from build123d import *

# Parameters (mm, degrees)
BOSS_EXTRUDE1_DEPTH = 10.16
FILLET1_R           = 19.05
SKETCH2_W           = 120.284747719
SKETCH2_H           = 20.32
SKETCH2_W_2         = 102.891608588
CUT_EXTRUDE1_DEPTH  = 12.7
SKETCH6_R           = 6.35
CUT_EXTRUDE2_DEPTH  = 10.16


with BuildPart() as part:
    # Sketch1 → Boss-Extrude1 (new body)
    with BuildSketch(Plane.XY):
        Polygon((-288.275887252, 0), (-215.032557346, 1054.1), (215.032557346, 1054.1), (288.275887252, 0), (596.950713016, 0), (596.950713016, 20.32), (457.769290722, 178.8375841), (368.537470958, 1463.04), (215.892500906, 1463.04), (-205.715298803, 1463.040000035), (-647.718210796, 1463.04), (-647.718210796, 0), align=None)
        Polygon((-609.618210796, 127), (-609.618210796, 461.510956689), (-365.626284392, 127), align=None, mode=Mode.SUBTRACT)
        Polygon((-609.618210796, 592.582701044), (-609.618210796, 907.626666667), (-314.736774564, 907.626666667), align=None, mode=Mode.SUBTRACT)
        Polygon((-282.735998162, 867.476761947), (-304.419486117, 555.413333333), (-574.827649063, 555.413333333), align=None, mode=Mode.SUBTRACT)
        Polygon((-307.949285149, 504.613333333), (-331.453012037, 166.353473425), (-578.179384354, 504.613333333), align=None, mode=Mode.SUBTRACT)
        Polygon((-609.618210796, 958.426666667), (-609.618210796, 1288.067621407), (-310.704175954, 958.426666667), align=None, mode=Mode.SUBTRACT)
        Polygon((-575.330448642, 1325.88), (-250.884200804, 1325.88), (-273.976047339, 993.547820907), align=None, mode=Mode.SUBTRACT)
        Polygon((19.05, 1104.9), (19.05, 1368.504716774), (182.716004616, 1104.9), align=None, mode=Mode.SUBTRACT)
        Polygon((41.473134849, 1404.62), (184.313325179, 1404.62), (202.313466912, 1145.566384812), align=None, mode=Mode.SUBTRACT)
        Polygon((-184.313325179, 1404.62), (-41.473134849, 1404.62), (-202.313466912, 1145.566384812), align=None, mode=Mode.SUBTRACT)
        Polygon((-19.05, 1368.504716774), (-19.05, 1104.9), (-182.716004616, 1104.9), align=None, mode=Mode.SUBTRACT)
    extrude(amount=BOSS_EXTRUDE1_DEPTH)

    # Fillet1
    fillet1_edges = [part.edges().sort_by_distance(p)[0] for p in [
        (19.05, 1368.504716774, 5.08),
        (19.05, 1104.9, 5.08),
        (182.716004616, 1104.9, 5.08),
        (-250.884200804, 1325.88, 5.08),
        (-575.330448642, 1325.88, 5.08),
        (-273.976047339, 993.547820907, 5.08),
        (-647.718210796, 1463.04, 5.08),
        (368.537470958, 1463.04, 5.08),
        (457.769290722, 178.8375841, 5.08),
        (215.032557346, 1054.1, 5.08),
        (-215.032557346, 1054.1, 5.08),
        (-609.618210796, 1288.067621407, 5.08),
        (-609.618210796, 958.426666667, 5.08),
        (-310.704175954, 958.426666667, 5.08),
        (-609.618210796, 461.510956689, 5.08),
        (-609.618210796, 127, 5.08),
        (-365.626284392, 127, 5.08),
        (-41.473134849, 1404.62, 5.08),
        (-184.313325179, 1404.62, 5.08),
        (-202.313466912, 1145.566384812, 5.08),
        (-182.716004616, 1104.9, 5.08),
        (-19.05, 1104.9, 5.08),
        (-19.05, 1368.504716774, 5.08),
        (184.313325179, 1404.62, 5.08),
        (41.473134849, 1404.62, 5.08),
        (202.313466912, 1145.566384812, 5.08),
        (-578.179384354, 504.613333333, 5.08),
        (-331.453012037, 166.353473425, 5.08),
        (-307.949285149, 504.613333333, 5.08),
        (-609.618210796, 907.626666667, 5.08),
        (-609.618210796, 592.582701044, 5.08),
        (-314.736774564, 907.626666667, 5.08),
        (-574.827649063, 555.413333333, 5.08),
        (-304.419486117, 555.413333333, 5.08),
        (-282.735998162, 867.476761947, 5.08),
    ]]
    fillet(fillet1_edges, radius=FILLET1_R)

    # Sketch2 → Cut-Extrude1 (cut)
    with BuildSketch(Plane.XY.offset(10.16)):
        with Locations((-467.291089218, 10.16)):
            Rectangle(SKETCH2_W, SKETCH2_H)
        with Locations((442.613300134, 10.16)):
            Rectangle(SKETCH2_W_2, SKETCH2_H)
        Polygon((211.92306481, 1373.664189215), (222.040744894, 1374.366931824), (215.881789204, 1463.040000035), (205.715298803, 1463.040000035), align=None)
        Polygon((234.358656272, 1197.020795404), (227.836927701, 1290.916856945), (217.719247617, 1290.214114336), (224.240976188, 1196.318052795), align=None)
        Polygon((246.676567651, 1019.674658983), (240.15668194, 1113.544188093), (230.039001856, 1112.841445484), (236.558887567, 1018.971916374), align=None)
        Polygon((258.99447903, 842.328522563), (252.476436179, 936.171519242), (242.358756095, 935.468776633), (248.876798945, 841.625779953), align=None)
        Polygon((271.312390408, 664.982386142), (264.796190418, 758.798850391), (254.678510334, 758.096107781), (261.194710324, 664.279643533), align=None)
        Polygon((283.630301787, 487.636249721), (277.115944656, 581.426181539), (266.998264572, 580.72343893), (273.512621703, 486.933507112), align=None)
        Polygon((295.948213166, 310.290113301), (289.435698895, 404.053512688), (279.318018811, 403.350770078), (285.830533081, 309.587370692), align=None)
        Polygon((308.266124544, 132.94397688), (301.755453134, 226.680843836), (291.63777305, 225.978101227), (298.14844446, 132.241234271), align=None)
        Polygon((-301.755453134, 226.680843836), (-308.266124544, 132.94397688), (-298.14844446, 132.241234271), (-291.63777305, 225.978101227), align=None)
        Polygon((-289.435698895, 404.053512688), (-295.948213166, 310.290113301), (-285.830533081, 309.587370692), (-279.318018811, 403.350770078), align=None)
        Polygon((-277.115944656, 581.426181539), (-283.630301787, 487.636249721), (-273.512621703, 486.933507112), (-266.998264572, 580.72343893), align=None)
        Polygon((-264.796190418, 758.798850391), (-271.312390408, 664.982386142), (-261.194710324, 664.279643533), (-254.678510334, 758.096107781), align=None)
        Polygon((-252.476436179, 936.171519242), (-258.99447903, 842.328522563), (-248.876798945, 841.625779953), (-242.358756095, 935.468776633), align=None)
        Polygon((-240.15668194, 1113.544188093), (-246.676567651, 1019.674658983), (-236.558887567, 1018.971916374), (-230.039001856, 1112.841445484), align=None)
        Polygon((-227.836927701, 1290.916856945), (-234.358656272, 1197.020795404), (-224.240976188, 1196.318052795), (-217.719247617, 1290.214114336), align=None)
        Polygon((-222.040744894, 1374.366931824), (-211.92306481, 1373.664189215), (-205.715298803, 1463.040000035), (-215.881789204, 1463.040000035), align=None)
    extrude(amount=-CUT_EXTRUDE1_DEPTH, mode=Mode.SUBTRACT)

    # Sketch6 → Cut-Extrude2 (cut)
    with BuildSketch(Plane.XY.offset(10.16)):
        with Locations((357.1875, 1397)):
            Circle(SKETCH6_R)
        with Locations((357.1875, 1320.8)):
            Circle(SKETCH6_R)
        with Locations((304.8, 1320.8)):
            Circle(SKETCH6_R)
        with Locations((304.8, 1397)):
            Circle(SKETCH6_R)
        with Locations((382.5875, 105.41)):
            Circle(SKETCH6_R)
        with Locations((382.5875, 29.21)):
            Circle(SKETCH6_R)
        with Locations((330.2, 29.21)):
            Circle(SKETCH6_R)
        with Locations((330.2, 105.41)):
            Circle(SKETCH6_R)
        with Locations((350.023844044, 410.21)):
            Circle(SKETCH6_R)
        with Locations((346.838891066, 562.61)):
            Circle(SKETCH6_R)
    extrude(amount=-CUT_EXTRUDE2_DEPTH, mode=Mode.SUBTRACT)


solid = part.part
Read the model definition and answer for the solid it produces. Units are mm, in the model's axes. A direction names the side the tool comes from. Round coordinates to 2 decimals unless told otherwise and drop trailing zeros. Order: outer loops, then holes, each group sorted by start corner. A loop starts at its lowest first (then second) coordinate and runs counter-clockwise, first axis right, second up. Notation, with made-up numbers: (-8.5, -40) - (-1.5, -40) arc R19 cw to (-1.5, -32) - close; hole circle Ø7 at (46, -3.75). An arc over 180 degrees is marked (long way). Use one line per item in the form item = value. Start each with the question number.
(1) For faces 1 (the face through (251.766, 525.44, 5.009)), 2 (the face through (-109.955, 1294.322, 5.009)), 3 (the face through (530.426, 96.087, 5.009)), determine the directions among +Z, -Z, +X, -X, +Y, -Y from which every point of the face is accessible in a straight line to the end or side of a thin tool.
(2) The part is cut by section A-A (y = 1353.5). Give the vertices of the cut face in (x, z).
(3) Flat-ended cylindrical pins translate along their axes: pin 1 Ø16.5 at (x, y) = (350.02, 410.21) entering from -Z; pin 2 Ø3 at (y, z) = (1135.5, 2.5) entering from +X; pin 3 Ø3 at (y, z) = (1256.5, 5) entering from +X; pin 4 Ø3 at (x, z) = (-432, 6.5) entering from -Y. Find the tip coordinate at first contact, or state that the pin passes through.
(4) Find the intervals of material crossed by line 1 along Y through (x, z) = (-593.5, 5); line 2 along Y through (x, z) = (330.2, 3.5); line 3 along X through (y, z) = (785.5, 9.5), in increasing order. Write a range as from..to.
(5) Determine the mould class of faces 4 (the face through (-252.774, 510.931, 5.009)), 5 (the face through (414.16, 806.46, 5.01)), 6 (the face through (-457.805, 339.581, 5.009)), 7 (the face through (-259, 897, 10.16)) for opening direction X: +X half, -X half, draft (parallel to the pull), parting line (faces both ways), or undercut.
(6) The part is cut by section B-B (z = 7). Count the separate pieces of the cut face and the enclosed holes in it, then the cut area to 3 significant figures.
Checked values:
q1.face_1 = +Z, -Z, -Y
q1.face_2 = +Z, -Z
q1.face_3 = +Z, -Z, +X, +Y
q2.outline = (-647.72, 0) - (-187.87, 0) - (-187.87, 10.16) - (-647.72, 10.16) - close; (-73.21, 0) - (73.21, 0) - (73.21, 10.16) - (-73.21, 10.16) - close; (187.87, 0) - (376.15, 0) - (376.15, 10.16) - (187.87, 10.16) - close
q3.pin_1 = 0
q3.pin_2 = 391.4
q3.pin_3 = 382.99
q3.pin_4 = 20.32
q4.line_1 = 0..127.23, 421.89..621.99, 907.4..958.65, 1257.52..1463.04
q4.line_2 = 0..22.86, 35.56..99.06, 111.76..1463.04
q4.line_3 = -647.72..-609.62, -429.05..-359.47, -288.43..-233.7, 233.7..415.62
q5.face_4 = undercut
q5.face_5 = +X half
q5.face_6 = undercut
q5.face_7 = draft
q6.separate_pieces = 1
q6.enclosed_holes = 34
q6.area = 675,000 mm^2
